Build history of the part. All positions in model axes, mm. Round coordinates to 2 decimals unless told otherwise and drop trailing zeros. Write each loop counter-clockwise with the first axis right and the second up, starting at its lowest first coordinate (ties: lowest second). Pieces come first, ordered by that corner, then holes.
Item 1: Band-saw the part on A-A, the plane y = 25. Write the cut outline in (x, z), then the cut area to 3 significant figures.
Item 2: Band-saw the part on D-D, the plane x = 27. Write the cut outline in (y, z).
Item 3: Drop flat-ended pins along their axis: pin 1 Ø13 at (x, y) = (0, 25) entering from -Z; pin 2 Ø1.5 at (x, z) = (11, 4) entering from +Y; pin 3 Ø1 at (x, z) = (-5, 3.5) entering from -Y. Give the stop position or say it passes through.
Item 4: Wall check: probe 1 along X at (y, z) = (-20, 3.8); probe 2 along X at (y, z) = (-12, 1.35); probe 3 along X at (y, z) = (2.5, 4.2). Give the ranges that are in metal, low to high.
Item 5: Mould opens along Y. For faces 1 (the flat face through (3, 11, 5)), 2 (the cylindrical face through (33.938, 3.512, 2.465)) say: +Y half, -Y half, draft (parallel to the pull), parting line (faces both ways), or undercut.
Item 6: Band-saw the part on C-C, the plane y = -26. Write the cut outline in (x, z).
Item 7: Band-saw the part on B-B, the plane x = -31. Write the cut outline in (y, z).
```python
from build123d import *

# Parameters (mm, degrees)
F0_R     = 11
F1_DEPTH = 5


with BuildPart() as f1:
    # F0 (on Top) → F1 (new body)
    with BuildSketch(Plane.XY):
        with BuildLine():
            ThreePointArc((8.228994, 11.326238), (7.290537, 11.951907), (6.30476, 12.5))
            ThreePointArc((6.30476, 12.5), (0, 39), (-6.30476, 12.5))
            ThreePointArc((-6.30476, 12.5), (-7.290537, 11.951907), (-8.228994, 11.326238))
            ThreePointArc((-8.228994, 11.326238), (-9.114039, 10.627055), (-9.939928, 9.858896))
            ThreePointArc((-9.939928, 9.858896), (-37.091204, 12.051663), (-13.836484, -2.133471))
            ThreePointArc((-13.836484, -2.133471), (-13.619838, -3.24037), (-13.314791, -4.326238))
            ThreePointArc((-13.314791, -4.326238), (-12.923323, -5.384026), (-12.447974, -6.406867))
            ThreePointArc((-12.447974, -6.406867), (-22.923625, -31.551663), (-2.246658, -13.818557))
            ThreePointArc((-2.246658, -13.818557), (-1.126986, -13.954566), (0, -14))
            ThreePointArc((0, -14), (1.126986, -13.954566), (2.246658, -13.818557))
            ThreePointArc((2.246658, -13.818557), (22.923625, -31.551663), (12.447974, -6.406867))
            ThreePointArc((12.447974, -6.406867), (12.923323, -5.384026), (13.314791, -4.326238))
            ThreePointArc((13.314791, -4.326238), (13.619838, -3.24037), (13.836484, -2.133471))
            ThreePointArc((13.836484, -2.133471), (37.091204, 12.051663), (9.939928, 9.858896))
            ThreePointArc((9.939928, 9.858896), (9.114039, 10.627055), (8.228994, 11.326238))
        make_face()
        with Locations((-14.694631, -20.225425)):
            Circle(F0_R, mode=Mode.SUBTRACT)
        with Locations((14.694631, -20.225425)):
            Circle(F0_R, mode=Mode.SUBTRACT)
        with BuildLine():
            ThreePointArc((-6.465638, 8.899187), (0, 11), (6.465638, 8.899187))
            ThreePointArc((6.465638, 8.899187), (10.461622, 3.399187), (10.461622, -3.399187))
            ThreePointArc((10.461622, -3.399187), (6.465638, -8.899187), (0, -11))
            ThreePointArc((0, -11), (-6.465638, -8.899187), (-10.461622, -3.399187))
            ThreePointArc((-10.461622, -3.399187), (-10.461622, 3.399187), (-6.465638, 8.899187))
        make_face(mode=Mode.SUBTRACT)
        with Locations((-23.776413, 7.725425)):
            Circle(F0_R, mode=Mode.SUBTRACT)
        with Locations((23.776413, 7.725425)):
            Circle(F0_R, mode=Mode.SUBTRACT)
        with Locations((0, 25)):
            Circle(F0_R, mode=Mode.SUBTRACT)
    extrude(amount=F1_DEPTH)


solid = f1.part
```
Results:
1. outline: (-14, 0) - (-11, 0) - (-11, 5) - (-14, 5) - close; (11, 0) - (14, 0) - (14, 5) - (11, 5) - close
1. area: 30.0 mm2
2. outline: (-26.9, 0) - (-13.55, 0) - (-13.55, 5) - (-26.9, 5) - close; (-5.9, 0) - (-2.79, 0) - (-2.79, 5) - (-5.9, 5) - close; (18.24, 0) - (21.35, 0) - (21.35, 5) - (18.24, 5) - close
3. pin 1: passes through
3. pin 2: stops at y = 34.54
3. pin 3: stops at y = -30.78
4. probe 1: x = -28.69 to -25.69, -3.7 to -0.7, 0.7 to 3.7, 25.69 to 28.69
4. probe 2: x = -26.02 to -22, -7.39 to 7.39, 22 to 26.02
4. probe 3: x = -36.76 to -33.46, -14.1 to -10.71, 10.71 to 14.1, 33.46 to 36.76
5. face 1: draft
5. face 2: undercut
6. outline: (-27.45, 0) - (-24.06, 0) - (-24.06, 5) - (-27.45, 5) - close; (-5.33, 0) - (-1.94, 0) - (-1.94, 5) - (-5.33, 5) - close; (1.94, 0) - (5.33, 0) - (5.33, 5) - (1.94, 5) - close; (24.06, 0) - (27.45, 0) - (27.45, 5) - (24.06, 5) - close
7. outline: (-4.27, 0) - (-0.57, 0) - (-0.57, 5) - (-4.27, 5) - close; (16.02, 0) - (19.72, 0) - (19.72, 5) - (16.02, 5) - close
